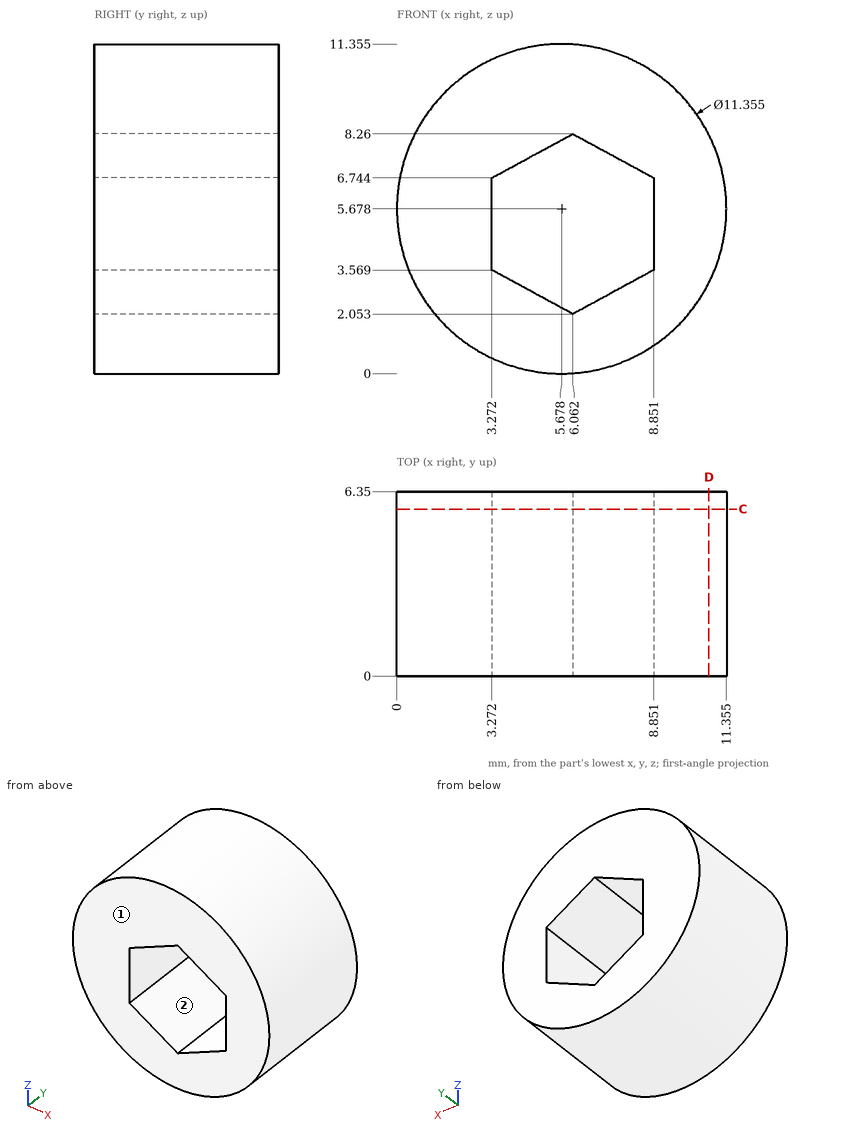
Can you work these out from the drawing? Everything is in mm from the part's minimum corner. A direction names the side the tool comes from. Round coordinates to 2 decimals unless told otherwise and drop trailing zeros. Loops run counter-clockwise (first coordinate to the right, second up) from the corner with the lowest first, then second, coordinate; pieces in that order, holes last. Notation, with made-up numbers: M 51.5,5 L 102.5,5 A24 ccw 102.5,21 Z; hole C 85.25,75 d5. An arc over 180 degrees is marked long. Write item = value, one per line.
1. Which directions (+Z, -Z, +X, -X, +Y, -Y) give clear straight access to the entire face, cutting with the end or side of a thin tool? Please do the marked faces 1 and 2.
Results below:
face_1 = +Z, -Z, +X, -X, -Y
face_2 = +Y, -Y
2. I want a section at D-D, the plane x = 10.75. Write out the boundary of the cut face in (y, z), and give its area (3 significant figures).
Results below:
outline = M 0,3.13 L 6.35,3.13 L 6.35,8.23 L 0,8.23 Z
area = 32.4 mm²
3. I want a section at C-C, the plane y = 5.75. Write out the boundary of the cut face in (x, z) (1 decimal).
Results below:
outline = C 5.7,5.7 d11.4; hole M 3.3,3.6 L 6.1,2.1 L 8.9,3.6 L 8.9,6.7 L 6.1,8.3 L 3.3,6.7 Z
4. I need wall thicknesses on probe 1 along Z at (x, y) = (4, 2.5) (1 decimal); probe 2 along Z at (x, y) = (8, 2.5) (1 decimal); probe 3 along X at (y, z) = (3.5, 3) (1 decimal). Which ranges of each line are inside material? Lowest first, please.
Results below:
probe_1 = 0.3 to 3.2, 7.1 to 11.1
probe_2 = 0.5 to 3.1, 7.2 to 10.9
probe_3 = 0.7 to 4.3, 7.8 to 10.7
5. Will these pins go through, and if not, where does the flat tip stop? P1, Ø1, axis at x = 8.5, y = 5, coming from the +Z side; P2, Ø2, axis at x = 3.5, y = 2.5, coming from the +Z side; P3, Ø3, axis at x = 1.5, y = 4, coming from the +Z side (1 decimal).
Results below:
P1 = 10.86
P2 = 11.23
P3 = 10.7
